Verification items for the finished model (mm, model axes). A direction names the side the tool comes from. Round coordinates to 2 decimals unless told otherwise and drop trailing zeros. Write each loop counter-clockwise with the first axis right and the second up, starting at its lowest first coordinate (ties: lowest second). Pieces come first, ordered by that corner, then holes. Notation, with made-up numbers: (36, -17.75) - (76, -17.75) arc R7 ccw to (76, -11.75) - close; hole circle Ø11 at (-23.5, 49). An arc over 180 degrees is marked (long way). Answer as a JSON object with one key per item and string values.
```python
from build123d import *

# Parameters (mm, degrees)
SKETCH1_R           = 30
SKETCH1_R_2         = 8.5
SKETCH1_R_3         = 3.4
BOSS_EXTRUDE1_DEPTH = 60
SKETCH3_R           = 30
SKETCH3_R_2         = 27.5
CUT_EXTRUDE1_DEPTH  = 5
CHAMFER1_SIZE       = 5


with BuildPart() as part:
    # Sketch1 → Boss-Extrude1 (new body)
    with BuildSketch(Plane(origin=(0, 0, 0), x_dir=(1, 0, 0), z_dir=(0, 1, 0))):
        Circle(SKETCH1_R)
        Circle(SKETCH1_R_2, mode=Mode.SUBTRACT)
        with Locations((-20, 0)):
            Circle(SKETCH1_R_3, mode=Mode.SUBTRACT)
        with Locations((0, 20)):
            Circle(SKETCH1_R_3, mode=Mode.SUBTRACT)
        with Locations((20, 0)):
            Circle(SKETCH1_R_3, mode=Mode.SUBTRACT)
        with Locations((0, -20)):
            Circle(SKETCH1_R_3, mode=Mode.SUBTRACT)
    extrude(amount=BOSS_EXTRUDE1_DEPTH)

    # Sketch3 → Cut-Extrude1 (cut)
    with BuildSketch(Plane(origin=(0, 60, 0), x_dir=(1, 0, 0), z_dir=(0, 1, 0))):
        Circle(SKETCH3_R)
        Circle(SKETCH3_R_2, mode=Mode.SUBTRACT)
    extrude(amount=-CUT_EXTRUDE1_DEPTH, mode=Mode.SUBTRACT)

    # Chamfer1
    chamfer1_edges = [part.edges().sort_by_distance(p)[0] for p in [
        (-8.5, 0, 0),
    ]]
    chamfer(chamfer1_edges, length=CHAMFER1_SIZE)


solid = part.part
```
1. Cross-section at A-A (z = 0). Record the boundary of the cut face in (x, y), plus the area to 3 significant figures.
Completed:
{"outline": "(-30, 0) - (-23.4, 0) - (-23.4, 60) - (-27.5, 60) - (-27.5, 55) - (-30, 55) - close; (-16.6, 0) - (-13.5, 0) - (-8.5, 5) - (-8.5, 60) - (-16.6, 60) - close; (8.5, 5) - (13.5, 0) - (16.6, 0) - (16.6, 60) - (8.5, 60) - close; (23.4, 0) - (30, 0) - (30, 55) - (27.5, 55) - (27.5, 60) - (23.4, 60) - close", "area": "1,710 mm^2"}
2. Cross-section at C-C (x = -22). Record the boundary of the cut face in (y, z), plus the area to 3 significant figures.
Completed:
{"outline": "(0, -20.4) - (55, -20.4) - (55, -16.5) - (60, -16.5) - (60, -2.75) - (0, -2.75) - close; (0, 2.75) - (60, 2.75) - (60, 16.5) - (55, 16.5) - (55, 20.4) - (0, 20.4) - close", "area": "2,080 mm^2"}
3. Cross-section at D-D (z = -20). Record the boundary of the cut face in (x, y).
Completed:
{"outline": "(-22.36, 0) - (-3.4, 0) - (-3.4, 60) - (-18.87, 60) - (-18.87, 55) - (-22.36, 55) - close; (3.4, 0) - (22.36, 0) - (22.36, 55) - (18.87, 55) - (18.87, 60) - (3.4, 60) - close"}
4. Access from +Z, -Z, +X, -X, +Y, -Y to the whole of each face (thin tool, end or side, straight path). Record for faces 1 (the face through (13.2, 55, 24.3)), 2 (the face through (-6.5, 60, 5.73)).
Completed:
{"face 1": "+Y", "face 2": "+Z, -Z, +X, -X, +Y"}
5. Material ranges on probe 1 along X at (y, z) = (31, 0); probe 2 along X at (y, z) = (9.5, -1); probe 3 along Z at (x, y) = (1.5, 28), recorded low to high. Write a range as from..to.
Completed:
{"probe 1": "x = -30..-23.4, -16.6..-8.5, 8.5..16.6, 23.4..30", "probe 2": "x = -29.98..-23.25, -16.75..-8.44, 8.44..16.75, 23.25..29.98", "probe 3": "z = -29.96..-23.05, -16.95..-8.37, 8.37..16.95, 23.05..29.96"}
6. Mould release check, pull along Z, two halves, no side actions. Record for faces 3 (the face through (-0.74, 29.58, 23.32)), 4 (the face through (6, 0, 13)), 5 (the face through (-5.961, 57.535, 26.846)): released by +Z, released by -Z, zero draft, split by the parting line, or undercut.
Completed:
{"face 3": "undercut", "face 4": "zero draft", "face 5": "split by the parting line"}
7. Go/stop test with flat-tipped pins: pin 1 (6 mm diameter, centred on y = 38, z = -3.5, fed in from +X); pin 2 (8 mm diameter, centred on x = -6.5, y = 52, fed in from +Z); pin 3 (6 mm diameter, centred on y = 9.5, z = -10.5, fed in from +X). Record where each tip stops, or that it passes through.
Completed:
{"pin 1": "stops at x = 30", "pin 2": "stops at z = 29.9", "pin 3": "stops at x = 29.05"}
8. Cross-section at B-B (x = 0). Record the boundary of the cut face in (y, z).
Completed:
{"outline": "(0, -30) - (55, -30) - (55, -27.5) - (60, -27.5) - (60, -23.4) - (0, -23.4) - close; (0, -16.6) - (60, -16.6) - (60, -8.5) - (5, -8.5) - (0, -13.5) - close; (0, 13.5) - (5, 8.5) - (60, 8.5) - (60, 16.6) - (0, 16.6) - close; (0, 23.4) - (60, 23.4) - (60, 27.5) - (55, 27.5) - (55, 30) - (0, 30) - close"}
